from build123d import *

# Parameters (mm, degrees)
BOSS_EXTRUDE1_DEPTH = 32
CUT_EXTRUDE1_REACH  = 146
SKETCH4_R           = 8
BOSS_EXTRUDE3_DEPTH = 22


with BuildPart() as part:
    # Sketch1 → Boss-Extrude1 (new body, symmetric)
    with BuildSketch(Plane.XY):
        Polygon((-72, 8), (-72, 28), (-56, 44), (-46, 44), (-46, 8), (72, 8), (72, -8), (-72, -8), align=None)
    extrude(amount=BOSS_EXTRUDE1_DEPTH, both=True)

    # Sketch2 → Cut-Extrude1 (cut, up to next)
    with BuildSketch(Plane(origin=(72, 0, 0), x_dir=(0, 0, -1), z_dir=(1, 0, 0)), mode=Mode.PRIVATE) as cut_extrude1_sk1:
        Polygon((-16, -8), (-16, -1), (-8, -1), (-8, 8), (8, 8), (8, -1), (16, -1), (16, -8), align=None)
    cut_extrude1_tool1 = extrude(cut_extrude1_sk1.sketch, amount=-CUT_EXTRUDE1_REACH, mode=Mode.PRIVATE) & part.part
    add(cut_extrude1_tool1.solids().sort_by_distance((72, -1.369565, 0))[0], mode=Mode.SUBTRACT)

    # Sketch4 → Boss-Extrude3 (add)
    with BuildSketch(Plane(origin=(72, 0, 0), x_dir=(0, 0, -1), z_dir=(1, 0, 0))):
        with BuildLine():
            Line((-14.476806191, 34.813375266), (-26.285598839, 9.722492138))
            ThreePointArc((-26.285598839, 9.722492138), (-27.392598928, 8.466965892), (-29, 8))
            Line((-29, 8), (29, 8))
            ThreePointArc((29, 8), (27.392598928, 8.466965892), (26.285598839, 9.722492138))
            Line((26.285598839, 9.722492138), (14.476806191, 34.813375266))
            ThreePointArc((14.476806191, 34.813375266), (0, 44), (-14.476806191, 34.813375266))
        make_face()
        with Locations((0, 28)):
            Circle(SKETCH4_R, mode=Mode.SUBTRACT)
    extrude(amount=-BOSS_EXTRUDE3_DEPTH)


solid = part.part
CAD build for the part. Positions are in the model's coordinates, mm. A direction names the side the tool comes from. Round coordinates to 2 decimals unless told otherwise and drop trailing zeros. Loops run counter-clockwise (first coordinate to the right, second up) from the corner with the lowest first, then second, coordinate; pieces in that order, holes last. Notation, with made-up numbers: (7, 22) - (18, 22) arc R20 cw to (18, 30) - close; hole circle Ø3 at (6.5, 60.25). An arc over 180 degrees is marked (long way). Put each result on its own line as item: value.
1. Two-plate mould, pull along Y, no slides. Class faces 5 (the flat face through (1, 4, -8)), 6 (the cylindrical face through (61.154, 35.932, 1.041)), 7 (the flat face through (61.154, 22.092, -20.464)), 8 (the flat face through (61, 8, 0)): released by +Y, released by -Y, zero draft, split by the parting line, or undercut.
Geometry check:
face 5: zero draft
face 6: undercut
face 7: released by +Y
face 8: released by -Y
2. 3-axis set-ups, long thin cutter, end or side, ignore diameter. For faces 1 (the flat face through (50, 18, 0)), 2 (the flat face through (1, -4, -16)), 3 (the cylindrical face through (61.154, 8.454, -27.413)), 4 (the flat face through (61.15, 22.44, 20.3)): which of +Z, -Z, +X, -X, +Y, -Y reach the whole face in a straight line?
Geometry check:
face 1: +Z, -Z, +Y
face 2: +X, -X, -Y
face 3: -Z, +X, +Y
face 4: +Z, +X, +Y
3. Slice it at C-C on x = -37. List the corners of the cut face in (y, z), and give its area (3 significant figures).
Geometry check:
outline: (-8, -32) - (8, -32) - (8, -8) - (-1, -8) - (-1, -16) - (-8, -16) - close; (-8, 16) - (-1, 16) - (-1, 8) - (8, 8) - (8, 32) - (-8, 32) - close
area: 656 mm²
4. Pin check, flat tips, straight feed: P1, Ø8, axis at x = 37.5, z = 6, coming from the -Y side; P2, Ø19, axis at x = 24.5, z = 14.5, coming from the +Y side; P3, Ø1, axis at x = 48, y = 9.5, coming from the +Z side; P4, Ø8, axis at x = -58, z = -2.5, coming from the -Y side. Stop position of each tip, or through.
Geometry check:
P1: y = -1
P2: y = 8
P3: through
P4: y = 8
5. Wall check: line 1 (X direction, y = 10, z = 16); line 2 (Z direction, x = 9.5, y = 0); line 3 (X direction, y = 26.5, z = -27). Give the ranges that are in metal, low to high.
Geometry check:
line 1: -72 to -46, 50 to 72
line 2: -32 to -8, 8 to 32
line 3: -72 to -46
6. Slice it at D-D on y = 32. List the corners of the cut face in (x, z), and give its area (3 significant figures).
Geometry check:
outline: (-68, -32) - (-46, -32) - (-46, 32) - (-68, 32) - close; (50, -15.8) - (72, -15.8) - (72, -6.93) - (50, -6.93) - close; (50, 6.93) - (72, 6.93) - (72, 15.8) - (50, 15.8) - close
area: 1,800 mm²
7. Slice it at A-A on z = 0. List the corners of the cut face in (x, y), and give its area (3 significant figures).
Geometry check:
outline: (-72, 8) - (-46, 8) - (-46, 44) - (-56, 44) - (-72, 28) - close; (50, 8) - (72, 8) - (72, 20) - (50, 20) - close; (50, 36) - (72, 36) - (72, 44) - (50, 44) - close
area: 1,250 mm²
8. Slice it at B-B on y = 5. List the corners of the cut face in (x, z).
Geometry check:
outline: (-72, -32) - (72, -32) - (72, -8) - (-72, -8) - close; (-72, 8) - (72, 8) - (72, 32) - (-72, 32) - close
